Job drawing, mm, ordinate dimensions from the low corner. One solid piece. Coordinates: 2 decimals unless noted, no trailing zeros. Order: outer loops, then holes, each group sorted by start corner. A loop starts at its lowest first (then second) coordinate and runs counter-clockwise, first axis right, second up. Notation, with made-up numbers: (76.25, 31) - (120.25, 31) arc R20 ccw to (120.25, 49) - close; hole circle Ø6 at (37.5, 49.5). An arc over 180 degrees is marked (long way). Use a Markdown table: item, result. Add a question column.
1) Wall check: L1, parallel to Z at x = 9.5, y = 1.75; L2, parallel to X at y = 2.5, z = 6; L3, parallel to Y at x = 11.25, z = 22. Give the ranges that are in metal, low to high. Write a range as [from, to].
2) Two-plate mould, pull along X, no slides. Class the marked faces 1, 2, 3 and 4: +X half, -X half, draft (parallel to the pull), parting line (faces both ways), or undercut.
3) Saw through at D-D on x = 1.5. List the corners of the cut face in (y, z).
4) Saw through at B-B on x = 8.5. List the corners of the cut face in (y, z), then the cut area to 3 significant figures.
5) Drop flat-ended pins along their axis: P1, Ø0.8, axis at x = 10, z = 0.5, coming from the +Y side; P2, Ø8, axis at x = 10, y = 9.5, coming from the -Z side. Give the stop position or say it passes through.
6) Saw through at C-C on z = 11.5. List the corners of the cut face in (x, y).
7) Saw through at A-A on y = 9. List the corners of the cut face in (x, z), then the cut area to 3 significant figures.
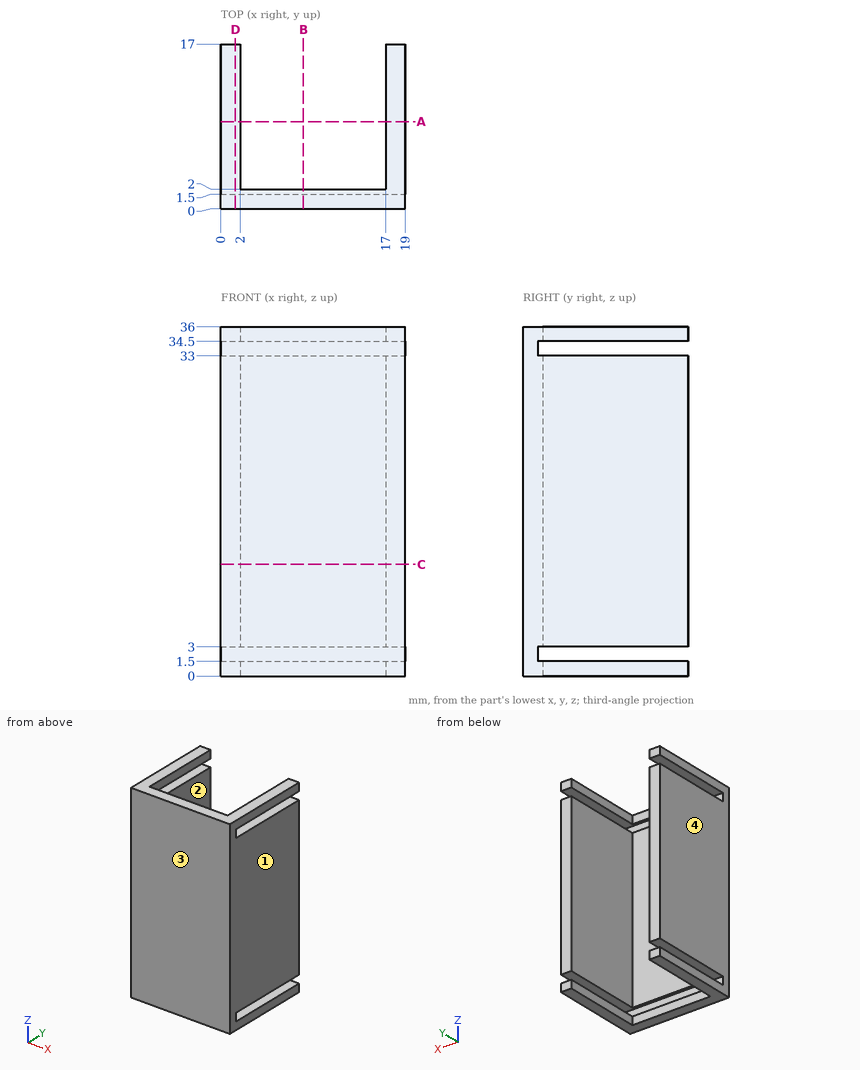
Results are:
| question | item | result |
|---|---|---|
| 1 | L1 | [0, 1.5], [3, 33], [34.5, 36] |
| 1 | L2 | [0, 2], [17, 19] |
| 1 | L3 | [0, 2] |
| 2 | face 1 | +X half |
| 2 | face 2 | undercut |
| 2 | face 3 | draft |
| 2 | face 4 | -X half |
| 3 | outline | (0, 0) - (17, 0) - (17, 1.5) - (1.5, 1.5) - (1.5, 3) - (17, 3) - (17, 33) - (1.5, 33) - (1.5, 34.5) - (17, 34.5) - (17, 36) - (0, 36) - close |
| 4 | outline | (0, 0) - (2, 0) - (2, 1.5) - (1.5, 1.5) - (1.5, 3) - (2, 3) - (2, 33) - (1.5, 33) - (1.5, 34.5) - (2, 34.5) - (2, 36) - (0, 36) - close |
| 4 | area | 70.5 mm2 |
| 5 | P1 | y = 2 |
| 5 | P2 | through |
| 6 | outline | (0, 0) - (19, 0) - (19, 17) - (17, 17) - (17, 2) - (2, 2) - (2, 17) - (0, 17) - close |
| 7 | outline | (0, 0) - (2, 0) - (2, 1.5) - (0, 1.5) - close; (0, 3) - (2, 3) - (2, 33) - (0, 33) - close; (0, 34.5) - (2, 34.5) - (2, 36) - (0, 36) - close; (17, 0) - (19, 0) - (19, 1.5) - (17, 1.5) - close; (17, 3) - (19, 3) - (19, 33) - (17, 33) - close; (17, 34.5) - (19, 34.5) - (19, 36) - (17, 36) - close |
| 7 | area | 132 mm2 |
